Autodesk Inventor part; units mm, degrees
ref_plane "YZ Plane" through (0, 0, 0) normal (1, 0, 0) x (0, 1, 0)
ref_plane "XZ Plane" through (0, 0, 0) normal (0, 1, 0) x (-1, 0, 0)
ref_plane "XY Plane" through (0, 0, 0) normal (0, 0, 1) x (1, 0, 0)
sketch "Sketch1" plane through (0, 0, 0) normal (0, 1, 0) x (-1, 0, 0)
  line L0 (-2.439, 103.9756) -> (-2.439, -118.4634)
  line L1 (89.878, -0.9024) -> (-81.0976, -0.9024)
  line L2 (87.561, 12.0976) -> (42.561, 12.0976)
  line L3 (42.561, 12.0976) -> (42.561, -13.9024)
  line L4 (42.561, -13.9024) -> (87.561, -13.9024)
  line L5 (87.561, -13.9024) -> (87.561, 12.0976)
  line L6 (31.3026, 83.5398) -> (8.8026, 44.5687)
  line L7 (8.8026, 44.5687) -> (31.3193, 31.5687)
  line L8 (31.3193, 31.5687) -> (53.8193, 70.5398)
  line L9 (53.8193, 70.5398) -> (31.3026, 83.5398)
  line L10 (-58.6974, 70.5398) -> (-36.1974, 31.5687)
  line L11 (-36.1974, 31.5687) -> (-13.6807, 44.5687)
  line L12 (-13.6807, 44.5687) -> (-36.1807, 83.5398)
  line L13 (-36.1807, 83.5398) -> (-58.6974, 70.5398)
  line L14 (-92.439, -13.9024) -> (-47.439, -13.9024)
  line L15 (-47.439, -13.9024) -> (-47.439, 12.0976)
  line L16 (-47.439, 12.0976) -> (-92.439, 12.0976)
  line L17 (-92.439, 12.0976) -> (-92.439, -13.9024)
  line L18 (-36.1807, -85.3447) -> (-13.6807, -46.3736)
  line L19 (-13.6807, -46.3736) -> (-36.1974, -33.3736)
  line L20 (-36.1974, -33.3736) -> (-58.6974, -72.3447)
  line L21 (-58.6974, -72.3447) -> (-36.1807, -85.3447)
  line L22 (53.8193, -72.3447) -> (31.3193, -33.3736)
  line L23 (31.3193, -33.3736) -> (8.8026, -46.3736)
  line L24 (8.8026, -46.3736) -> (31.3026, -85.3447)
  line L25 (31.3026, -85.3447) -> (53.8193, -72.3447)
  point P0 (0, 0)
  point P1 (-2.439, -0.9024)
  point P2 (43.7195, 79.0465)
  point P3 (-48.5976, 79.0465)
  point P4 (-94.7561, -0.9024)
  point P5 (-48.5976, -80.8514)
  point P6 (43.7195, -80.8514)
  dimension "d0" = 180
  dimension "d1" = 26
  dimension "d3" = 90
  dimension "d6" = 360
extrude "Extrusion1" add sketch "Sketch1" along normal blind 20
sketch "Sketch2" plane through (-8.8026, 0, -46.3736) normal (0.5, 0, 0.866) x (0.866, 0, -0.5)
  line L0 (-26, 0) -> (0, 0)
  line L1 (0, 0) -> (0, 20)
  line L2 (-26, 20) -> (0, 20)
  line L3 (-26, 0) -> (-26, 20)
  line L4 (-23, 23) -> (0, 0)
  line L5 (-26, 20) -> (0, 20)
  line L6 (-23, -3) -> (0, 20)
  point P0 (-15.5635, 0)
  point P1 (-11.6957, 8.3043)
extrude "Extrusion2" [suppressed]
pattern_circular "Circular Pattern1" [suppressed]
ref_plane "Work Plane1" through (24.939, 0, -39.8736) normal (-0.866, 0, -0.5) x (-0.5, 0, 0.866)
sketch "Sketch3" plane through (24.939, 0, -39.8736) normal (-0.866, 0, -0.5) x (-0.5, 0, 0.866)
  line L0 (45, 26.4) -> (45, -4.4)
  line L1 (0, 20) -> (-50, 20)
  line L2 (-50, 20) -> (-50, 22)
  line L3 (-50, 22) -> (0, 22)
  line L4 (0, 22) -> (0, 20)
  line L5 (-11.2583, 20) -> (11.2583, 20)
  point P0 (47.001, 0)
  dimension "d16" = 90
  dimension "d18" = 2
  dimension "d19" = 0
  dimension "d21" = 190
revolve "Revolution1" add sketch "Sketch3" angle 360 about axis through (2.439, 0, -0.9024) along (0, -1, 0)
properties part number "rotor-type2"
Can you work these out from the model? Positions are in its coordinate system, mm. A direction names the side the tool comes from. Give positions to 0.01 mm unless a question says otherwise; leave off trailing zeros. Loops run counter-clockwise (first coordinate to the right, second up) from the corner with the lowest first, then second, coordinate; pieces in that order, holes last. Notation, with made-up numbers: (-22.75, 37.5) - (-13.75, 37.5) arc R21 ccw to (-13.75, 48.5) - close; hole circle Ø1 at (53.5, -37). An arc over 180 degrees is marked (long way). Answer as a JSON object with one key per item and string values.
Q1. Which directions (+Z, -Z, +X, -X, +Y, -Y) give clear straight access to the entire face, cutting with the end or side of a thin tool? Please do faces 1 (the flat face through (24.773, 9.86, 63.781)), 2 (the flat face through (-19.895, 9.86, -65.586)), 3 (the flat face through (-87.561, 10, -1)), 4 (the flat face through (-42.72, 9.86, 76.95)), 5 (the flat face through (47.439, 10, -1)).
Geometry says:
{"face 1": "+Z, -Y", "face 2": "-Z, -Y", "face 3": "+Z, -Z, -X, -Y", "face 4": "+Z, -X, -Y", "face 5": "-Y"}
Q2. Imagine slicing it at D-D on x = 62.5. Write out the boundary of the cut face in (y, z), plus the area to 3 significant figures.
Geometry says:
{"outline": "(0, -13.9) - (20, -13.9) - (20, -74.51) - (22, -74.51) - (22, 72.7) - (20, 72.7) - (20, 12.1) - (0, 12.1) - close", "area": "814 mm²"}
Q3. If I drill on L1, parallel to Z at x = 54, y = 8.5; L2, parallel to Y at x = 25, z = -87; L3, parallel to Z at x = -75, y = 4.25, over which ranges is the centre line in solid material (lowest first)?
Geometry says:
{"L1": "-75.06 to -64.21, -13.9 to 12.1, 62.4 to 73.25", "L2": "20 to 22", "L3": "-13.9 to 12.1"}
Q4. Imagine slicing it at C-C on x = 1. Write out the boundary of the cut face in (y, z).
Geometry says:
{"outline": "(20, -95.89) - (22, -95.89) - (22, -45.88) - (20, -45.88) - close; (20, 44.07) - (22, 44.07) - (22, 94.09) - (20, 94.09) - close"}
Q5. If we mould it in two halves opening along X, with no side actions, what happens to faces 6 (the cylindrical face through (97.347, 21.014, 3.275)), 7 (the flat face through (47.3, 9.9, -52.6)), 8 (the flat face through (6, 20, -46))? For each: pulls with the +X half, pulls with the -X half, needs draft (parallel to the pull), parting line crosses it, or undercut.
Geometry says:
{"face 6": "parting line crosses it", "face 7": "pulls with the +X half", "face 8": "undercut"}
Q6. Imagine slicing it at A-A on y = 11.75. Write out the boundary of the cut face in (x, z), plus the area to 3 significant figures.
Geometry says:
{"outline": "(-87.56, -13.9) - (-42.56, -13.9) - (-42.56, 12.1) - (-87.56, 12.1) - close; (-53.82, -72.34) - (-31.3, -85.34) - (-8.8, -46.37) - (-31.32, -33.37) - close; (-53.82, 70.54) - (-31.32, 31.57) - (-8.8, 44.57) - (-31.3, 83.54) - close; (13.68, -46.37) - (36.18, -85.34) - (58.7, -72.34) - (36.2, -33.37) - close; (13.68, 44.57) - (36.2, 31.57) - (58.7, 70.54) - (36.18, 83.54) - close; (47.44, -13.9) - (92.44, -13.9) - (92.44, 12.1) - (47.44, 12.1) - close", "area": "7,020 mm²"}
Q7. Will these pins go through, and if not, where does the flat tip stop? P1, Ø10, axis at x = 31, y = 7, coming from the -Z side; P2, Ø6, axis at x = 22, y = 17.5, coming from the -Z side; P3, Ø10, axis at y = 7.5, z = -39, coming from the -X side.
Geometry says:
{"P1": "z = -85.03", "P2": "z = -94.2", "P3": "x = -37.45"}
Q8. Imagine slicing it at B-B on z = 40.5. Write out the boundary of the cut face in (x, y).
Geometry says:
{"outline": "(-83.06, 20) - (-36.48, 20) - (-36.48, 0) - (-15.85, 0) - (-15.85, 20) - (-15.19, 20) - (-15.19, 22) - (-83.06, 22) - close; (20.07, 20) - (20.73, 20) - (20.73, 0) - (41.35, 0) - (41.35, 20) - (87.94, 20) - (87.94, 22) - (20.07, 22) - close"}
